Source: CAD feature listing. Evaluate the final solid. Frame: model axes, mm. A direction names the side the tool comes from. Coordinates: 2 decimals unless noted, no trailing zeros. Loops run counter-clockwise (first coordinate to the right, second up) from the corner with the lowest first, then second, coordinate; pieces in that order, holes last. Notation, with made-up numbers: (-17, 80) -> (7, 80) arc R29 ccw to (7, 102) -> close; hole circle Ø7 at (-31.5, 87.5). An arc over 180 degrees is marked (long way). One line per question, with ' | ' between items. Start each with the question number.
```python
from build123d import *

# Parameters (mm, degrees)
F1_R     = 5
F1_R_2   = 2.15
F3_R     = 1
F5_DEPTH = 1.5


with BuildPart() as f2:
    # F2: sweep along a path in F0
    with BuildLine(Plane.XY) as f2_path:
        Line((0, 0), (-40, 0))
        ThreePointArc((-40, 0), (-54.1421356237, -5.8578643763), (-60, -20))
        Line((-60, -20), (-60, -60))
    # F1 (on Right) → F2 (sweep)
    with BuildSketch(Plane.YZ):
        Circle(F1_R)
        Circle(F1_R_2, mode=Mode.SUBTRACT)
    sweep(path=f2_path.line)

    # F3
    f3_edges = [f2.edges().sort_by_distance(p)[0] for p in [
        (-55, -60, 0),
        (0, -5, 0),
    ]]
    fillet(f3_edges, radius=F3_R)

    # F4 (on Top) → F5 (join, symmetric)
    with BuildSketch(Plane.XY):
        Polygon((-19.8250226729, 5), (-20, 3), (-6, 3), (-6.1749773271, 5), align=None)
        with BuildLine():
            Line((-19.634795067, 7.1743114855), (-19.8250226729, 5))
            Line((-19.8250226729, 5), (-6.1749773271, 5))
            Line((-6.1749773271, 5), (-6.365204933, 7.1743114855))
            ThreePointArc((-6.365204933, 7.1743114855), (-7.006413914, 8.4745546736), (-8.3575943292, 9))
            Line((-8.3575943292, 9), (-17.6424056708, 9))
            ThreePointArc((-17.6424056708, 9), (-18.993586086, 8.4745546736), (-19.634795067, 7.1743114855))
        make_face()
        with BuildLine():
            Line((-8.3575943292, 6), (-17.6424056708, 6))
            ThreePointArc((-17.6424056708, 6), (-18.6424056708, 7), (-17.6424056708, 8))
            Line((-17.6424056708, 8), (-8.3575943292, 8))
            ThreePointArc((-8.3575943292, 8), (-7.3575943292, 7), (-8.3575943292, 6))
        make_face(mode=Mode.SUBTRACT)
    extrude(amount=F5_DEPTH, both=True)


solid = f2.part
```
(1) Contact query for flat-ended pins moving along their axis: pin 1 Ø3.5 at (x, y) = (-15.5, 8) entering from -Z; pin 2 Ø5 at (x, z) = (-19, -2.5) entering from +Y; pin 3 Ø1.5 at (x, z) = (-44.5, 0.5) entering from +Y; pin 4 Ø1.5 at (y, z) = (-44.5, 2) entering from -X. Output: stop coordinate, or through.
(2) Draft query along X for faces 4 (the flat face through (-13, 8, 0)), 5 (the flat face through (-13, 6, 0)), 6 (the cylindrical face through (-6.99, 8.46, 0.02)), 7 (the flat face through (-13.1, 5.5, 1.5)). Return one class per face: pulls with the +X half, pulls with the -X half, needs draft (parallel to the pull), parting line crosses it, or undercut.
(3) Cut plane A-A, the plane x = -25.5. Return the cut outline in (y, z).
(4) Ray query, L1, parallel to Y at x = -28, z = 0; L2, parallel to X at y = -35.5, z = 0. Return the intervals inside material, ascending.
(5) Cut plane B-B, the plane y = -41. Return the cut outline in (x, z).
(6) Access query for faces 1 (the cylindrical face through (-20.28, -2.15, -0.09)), 2 (the cylindrical face through (-7.358, 7.022, 0.021)), 3 (the cylindrical face through (-55, -40, 0)). Directions: +Z, -Z, +X, -X, +Y, -Y. A direction counts if a zero-diameter tool reaches every point of the face in a straight line with its end or side. Return the directions, or none.
Here are the results:
1) pin 1: stops at z = -1.5 | pin 2: stops at y = 9 | pin 3: stops at y = 4.7 | pin 4: stops at x = -64.84
2) face 4: undercut | face 5: undercut | face 6: pulls with the +X half | face 7: needs draft
3) outline: circle Ø10 at (0, 0); hole circle Ø4.3 at (0, 0)
4) L1: y = -5 to -2.15, 2.15 to 5 | L2: x = -65 to -62.15, -57.85 to -55
5) outline: circle Ø10 at (-60, 0); hole circle Ø4.3 at (-60, 0)
6) face 1: +X | face 2: +Z, -Z | face 3: -Y
